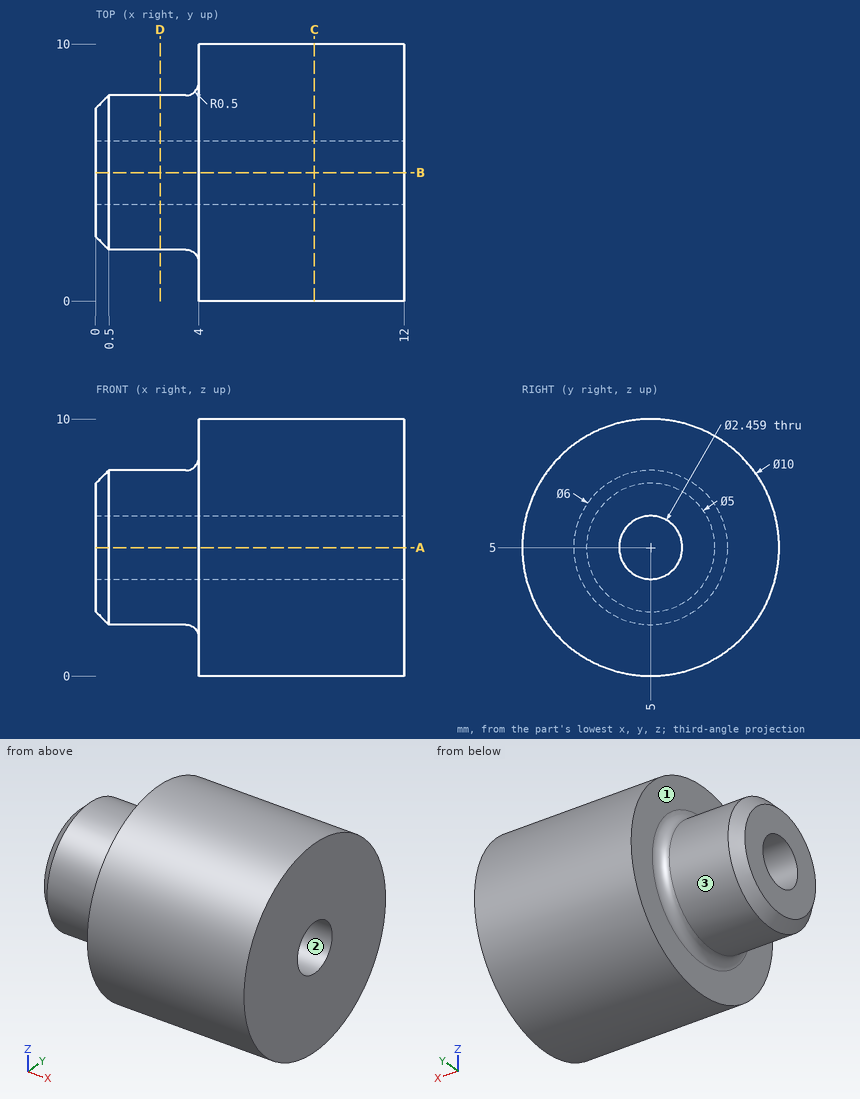
Input: dimensioned drawing with shaded views. Units: mm. Origin: part minimum x, y, z. Give positions to 0.01 mm unless a question says otherwise; leave off trailing zeros. Write each loop counter-clockwise with the first axis right and the second up, starting at its lowest first coordinate (ties: lowest second). Pieces come first, ordered by that corner, then holes. Notation, with made-up numbers: M -29.75,52 L 22.25,52 A12 cw 22.25,58 Z; hole C -24,34.5 d2. An arc over 180 degrees is marked long. Return JSON: item names as keys, results as strings. Group by question number.
1) Cut plane A-A, the plane z = 5. Output: boundary loops of the cut face in (x, y), plus the area to 3 significant figures.
2) Cut plane D-D, the plane x = 2.5. Output: boundary loops of the cut face in (y, z).
3) Pull-direction query (Y, two-part tool) for the marked faces 1, 2 and 3; classes: pulls with the +Y half, pulls with the -Y half, needs draft (parallel to the pull), parting line crosses it, or undercut.
4) Material intervals for line 1 along Z through (x, y) = (5.25, 5); line 2 along X through (y, z) = (5.25, 0.5); line 3 along Z through (x, y) = (7, 5.75), sorted ascending. Write a range as [from, to].
5) Pin query (flat end, axial travel): P1, Ø4, axis at x = 6.5, z = 2, coming from the +Y side; P2, Ø1.5, axis at x = 5.5, z = 8.5, coming from the +Y side. Return the tip coordinate at first contact, or that it passes through.
6) Cut plane C-C, the plane x = 8.5. Output: boundary loops of the cut face in (y, z).
Recorded:
{
 "1": {"outline": "M 0,2.5 L 0.5,2 L 3.5,2 A0.5 cw 4,1.5 L 4,0 L 12,0 L 12,3.77 L 0,3.77 Z; M 0,6.23 L 12,6.23 L 12,10 L 4,10 L 4,8.5 A0.5 cw 3.5,8 L 0.5,8 L 0,7.5 Z", "area": "74.3 mm²"},
 "2": {"outline": "C 5,5 d6; hole C 5,5 d2.46"},
 "3": {"face 1": "needs draft", "face 2": "undercut", "face 3": "parting line crosses it"},
 "4": {"line 1": "z = [0, 3.77], [6.23, 10]", "line 2": "x = [4, 12]", "line 3": "z = [0.06, 4.03], [5.97, 9.94]"},
 "5": {"P1": "stops at y = 9.9", "P2": "stops at y = 9.18"},
 "6": {"outline": "C 5,5 d10; hole C 5,5 d2.46"}
}
